Geometry check sheet. Reference: drawing and pictorial views, mm from the part's lowest x, y, z. Give positions to 0.01 mm unless a question says otherwise; leave off trailing zeros. Write each loop counter-clockwise with the first axis right and the second up, starting at its lowest first coordinate (ties: lowest second). Pieces come first, ordered by that corner, then holes. Notation, with made-up numbers: M -30.75,75.25 L 21.25,75.25 A33 ccw 21.25,106.25 Z; hole C -29,7 d8. An arc over 180 degrees is marked long. One line per item, written item: value. Start each with the question number.
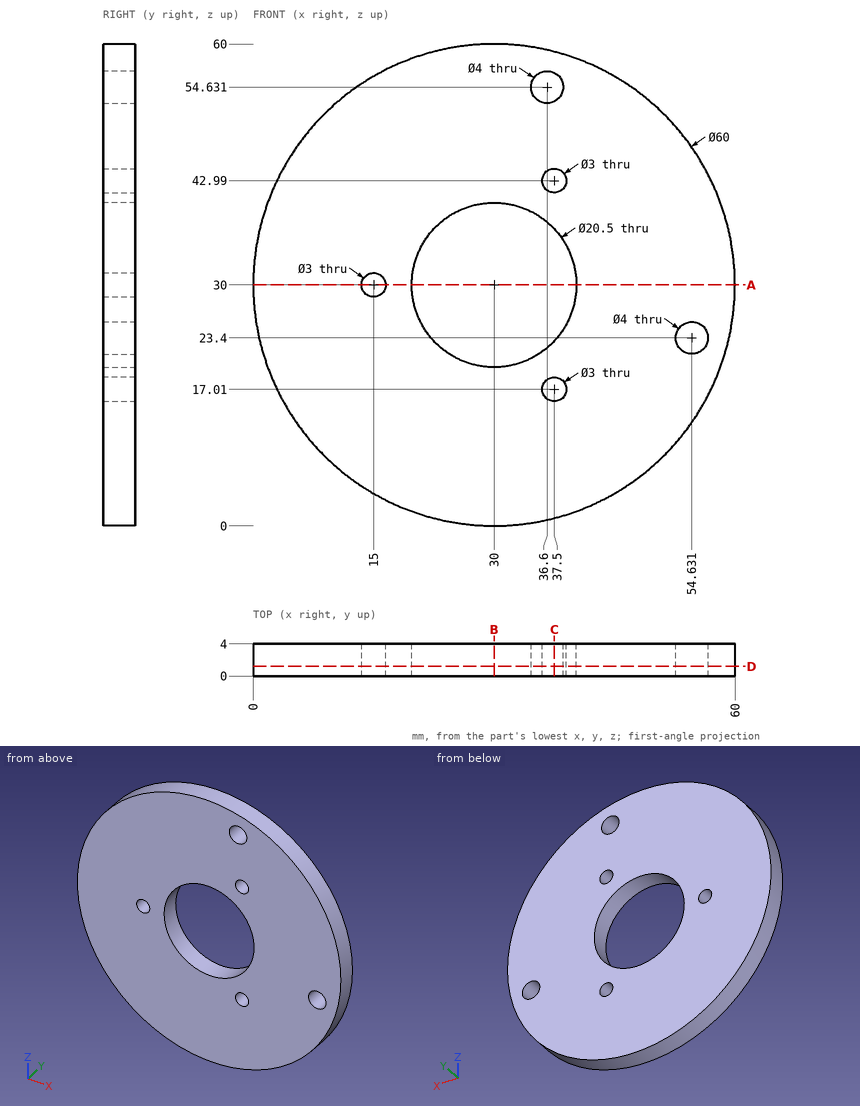
1) Cross-section at C-C (x = 37.5). Record the boundary of the cut face in (y, z) (1 decimal).
2) Cross-section at B-B (x = 30). Record the boundary of the cut face in (y, z), plus the area to 3 significant figures.
3) Cross-section at D-D (y = 1.2). Record the boundary of the cut face in (x, z), plus the area to 3 significant figures.
4) Gauge pin test, flat ends, axial feed: pin 1 (2 mm diameter, centred on y = 2.5, z = 9, fed in from +X); pin 2 (2 mm diameter, centred on y = 2.5, z = 23.5, fed in from -X). Record the tip position at first contact, or that the pin passes through.
5) Cross-section at A-A (z = 30). Record the boundary of the cut face in (x, y).
6) Material ranges on L1, parallel to X at y = 3.55, z = 22 (1 decimal); L2, parallel to X at y = 1.65, z = 39 (1 decimal); L3, parallel to X at y = 1.9, z = 36 (1 decimal), recorded low to high. Write a range as from..to.
Data:
1. outline: M 0,1 L 4,1 L 4,15.5 L 0,15.5 Z; M 0,18.5 L 4,18.5 L 4,23 L 0,23 Z; M 0,37 L 4,37 L 4,41.5 L 0,41.5 Z; M 0,44.5 L 4,44.5 L 4,52.8 L 0,52.8 Z; M 0,56.4 L 4,56.4 L 4,59 L 0,59 Z
2. outline: M 0,0 L 4,0 L 4,19.75 L 0,19.75 Z; M 0,40.25 L 4,40.25 L 4,60 L 0,60 Z
2. area: 158 mm2
3. outline: C 30,30 d60; hole C 15,30 d3; hole C 30,30 d20.5; hole C 36.6,54.63 d4; hole C 37.5,17.01 d3; hole C 37.5,42.99 d3; hole C 54.63,23.4 d4
3. area: 2,450 mm2
4. pin 1: stops at x = 52.36
4. pin 2: stops at x = 0.51
5. outline: M 0,0 L 13.5,0 L 13.5,4 L 0,4 Z; M 16.5,0 L 19.75,0 L 19.75,4 L 16.5,4 Z; M 40.25,0 L 60,0 L 60,4 L 40.25,4 Z
6. L1: x = 1.1..23.6, 36.4..53.2, 56.1..58.9
6. L2: x = 1.4..25.1, 34.9..58.6
6. L3: x = 0.6..21.7, 38.3..59.4
